Part model, mm, in its own coordinate system. A direction names the side the tool comes from. Give positions to 0.01 mm unless a question says otherwise; leave off trailing zeros. Write each loop counter-clockwise with the first axis right and the second up, starting at its lowest first coordinate (ties: lowest second). Pieces come first, ordered by that corner, then holes.
```python
from build123d import *

# Parameters (mm, degrees)
BOSS_EXTRUDE1_DEPTH = 5
CUT_EXTRUDE2_DEPTH  = 8.048
SKETCH3_R           = 0.640852302
SKETCH3_R_2         = 0.683244838
CUT_EXTRUDE3_DEPTH  = 8.048


with BuildPart() as part:
    # Sketch1 → Boss-Extrude1 (new body)
    with BuildSketch(Plane(origin=(0, 0, 0), x_dir=(1, 0, 0), z_dir=(0, 1, 0))):
        with BuildLine():
            Line((-0.55984013, 25.079292929), (-35.890546419, 25.079292929))
            Line((-35.890546419, 25.079292929), (-35.890546419, 23.777222222))
            ThreePointArc((-35.890546419, 23.777222222), (-30.682904989, 11.204863653), (-18.110546419, 5.997222222))
            Line((-18.110546419, 5.997222222), (-17.78, 5.997222222))
            ThreePointArc((-17.78, 5.997222222), (-5.207641431, 0.789580792), (0, -11.782777778))
            Line((0, -11.782777778), (0, -15.913484848))
            ThreePointArc((0, -15.913484848), (5.207641431, -28.485843418), (17.78, -33.693484848))
            Line((17.78, -33.693484848), (77.312672268, -33.693484848))
            ThreePointArc((77.312672268, -33.693484848), (86.927320297, -30.869652248), (93.487957466, -23.295120763))
            Line((93.487957466, -23.295120763), (107.768626914, 7.997929157))
            ThreePointArc((107.768626914, 7.997929157), (108.308432376, 9.081526458), (108.920724009, 10.125878891))
            ThreePointArc((108.920724009, 10.125878891), (104.307418831, 41.01014517), (73.08061258, 40.926123744))
            ThreePointArc((73.08061258, 40.926123744), (69.142100225, 38.332807414), (64.660382122, 36.866051805))
            Line((64.660382122, 36.866051805), (2.680771994, 25.377106766))
            ThreePointArc((2.680771994, 25.377106766), (1.067293855, 25.153902931), (-0.55984013, 25.079292929))
        make_face()
    extrude(amount=BOSS_EXTRUDE1_DEPTH)

    # Sketch2 → Cut-Extrude2 (cut)
    with BuildSketch(Plane(origin=(0, 5, 0), x_dir=(1, 0, 0), z_dir=(0, 1, 0))):
        with BuildLine():
            Line((-18.110546419, 8.537222222), (-17.78, 8.537222222))
            ThreePointArc((-17.78, 8.537222222), (-3.411590206, 2.585632016), (2.54, -11.782777778))
            Line((2.54, -11.782777778), (2.54, -15.913484848))
            ThreePointArc((2.54, -15.913484848), (7.003692655, -26.689792194), (17.78, -31.153484848))
            Line((17.78, -31.153484848), (77.312672268, -31.153484848))
            ThreePointArc((77.312672268, -31.153484848), (85.55379915, -28.733056905), (91.177202437, -22.240601346))
            Line((91.177202437, -22.240601346), (105.457871886, 9.052448573))
            ThreePointArc((105.457871886, 9.052448573), (106.074792413, 10.290845489), (106.77455428, 11.484391127))
            ThreePointArc((106.77455428, 11.484391127), (102.651926694, 39.083763644), (74.746447235, 39.008678854))
            ThreePointArc((74.746447235, 39.008678854), (70.245290257, 36.044888763), (65.123326712, 34.368596639))
            Line((65.123326712, 34.368596639), (3.143716583, 22.879651599))
            ThreePointArc((3.143716583, 22.879651599), (1.299741567, 22.624561503), (-0.55984013, 22.539292929))
            Line((-0.55984013, 22.539292929), (-33.300185357, 22.539292929))
            ThreePointArc((-33.300185357, 22.539292929), (-28.439911298, 12.571785095), (-18.110546419, 8.537222222))
        make_face()
    extrude(amount=-CUT_EXTRUDE2_DEPTH, mode=Mode.SUBTRACT)

    # Sketch3 → Cut-Extrude3 (cut)
    with BuildSketch(Plane(origin=(0, 5, 0), x_dir=(1, 0, 0), z_dir=(0, 1, 0))):
        with Locations(Location((-30.261155499, 24.077194613, 0), (0, 0, 270))):
            Circle(SKETCH3_R)
        with Locations(Location((103.209357625, 40.426722425, 0), (0, 0, 270))):
            Circle(SKETCH3_R_2)
    extrude(amount=-CUT_EXTRUDE3_DEPTH, mode=Mode.SUBTRACT)


solid = part.part
```
1) Pin check, flat tips, straight feed: pin 1 Ø1.1 at (x, z) = (103.21, -40.43) entering from -Y; pin 2 Ø3 at (x, y) = (59.5, 2.5) entering from -Z; pin 3 Ø1.2 at (y, z) = (3, 14.5) entering from +X. Stop position of each tip, or through.
Answers follow:
pin 1: passes through
pin 2: stops at z = -36.19
pin 3: stops at x = 97.78
2) Saw through at B-B, the plane z = 20. Write the cut outline in (x, y).
Answers follow:
outline: (0.48, 0) - (3.1, 0) - (3.1, 5) - (0.48, 5) - close; (92.2, 0) - (94.99, 0) - (94.99, 5) - (92.2, 5) - close
3) 3-axis set-ups, long thin cutter, end or side, ignore diameter. For faces 1 (the face through (0, 2, 14)), 2 (the face through (85.45, 2.54, 28.8)), 3 (the face through (-18, 2, -25.079)): which of +Z, -Z, +X, -X, +Y, -Y reach the whole face in a straight line?
Answers follow:
face 1: +Z, -X, +Y, -Y
face 2: +Y, -Y
face 3: -Z, -X, +Y, -Y
4) Two-plate mould, pull along X, no slides. Class faces 4 (the face through (38, 5, -31)), 5 (the face through (102.972, 2.535, -38.803)), 6 (the face through (5.07, 2.465, 28.347)): +X half, -X half, draft (parallel to the pull), parting line (faces both ways), or undercut.
Answers follow:
face 4: draft
face 5: undercut
face 6: -X half
5) Saw through at A-A, the plane x = 58. Write the cut outline in (y, z).
Answers follow:
outline: (0, -35.63) - (5, -35.63) - (5, -33.05) - (0, -33.05) - close; (0, 31.15) - (5, 31.15) - (5, 33.69) - (0, 33.69) - close
6) Wall check: L1, parallel to Z at x = 16.5, y = 2.9; L2, parallel to Z at x = -28, y = 1.6; L3, parallel to Z at x = 103.5, y = 1.3. Give the ranges that are in metal, low to high.
Answers follow:
L1: z = -27.94 to -25.36, 31.1 to 33.65
L2: z = -25.08 to -22.54, -12.18 to -9
L3: z = -41.67 to -41.05, -39.81 to -38.31, -4.76 to 1.36
7) Saw through at C-C, the plane y = 1. Count the separate pieces of the cut face and the enclosed holes in it, then the cut area to 3 significant figures.
Answers follow:
separate pieces: 1
enclosed holes: 3
area: 954 mm2
